Autodesk Inventor part; units mm, degrees
ref_plane "YZ Plane" through (0, 0, 0) normal (1, 0, 0) x (0, 1, 0)
ref_plane "XZ Plane" through (0, 0, 0) normal (0, 1, 0) x (-1, 0, 0)
ref_plane "XY Plane" through (0, 0, 0) normal (0, 0, 1) x (1, 0, 0)
sketch "Sketch1" plane through (0, 0, 0) normal (0, 1, 0) x (-1, 0, 0)
  line L0 (0, 0) -> (145, 0)
  line L1 (145, 0) -> (145, -145)
  line L2 (145, -145) -> (0, -145)
  line L3 (0, -145) -> (0, 0)
  dimension "d0" = 145
  dimension "d1" = 145
extrude "Extrusion1" add sketch "Sketch1" along normal blind 5
sketch "Sketch2" plane through (0, 5, 0) normal (0, 1, 0) x (1, 0, 0)
  line L0 (-145, 145) -> (-145, 0)
  line L1 (0, 145) -> (-145, 145)
  point P0 (0, 0)
  point P1 (-140, 72.5)
  dimension "d4" = 5
  dimension "d5" = 72.5
hole "Hole1" at (-140, 5, -72.5) direction (0, -1, 0) diameter 4 end through all
sketch "Sketch3" plane through (0, 5, 0) normal (0, 1, 0) x (1, 0, 0)
  line L0 (0, 0) -> (0, 145)
  line L1 (0, 145) -> (-145, 145)
  point P0 (-5, 72.5)
  dimension "d13" = 5
  dimension "d14" = 72.5
hole "Hole2" at (-5, 5, -72.5) direction (0, -1, 0) diameter 4 end through all
properties part number "pot_mover"
Build history of the part. All positions in model axes, mm. Round coordinates to 2 decimals unless told otherwise and drop trailing zeros. Loops run counter-clockwise (first coordinate to the right, second up) from the corner with the lowest first, then second, coordinate; pieces in that order, holes last.
Item 1: Saw through at B-B (z = -72.5). List the corners of the cut face in (x, y), then the cut area to 3 significant figures.
Item 2: Saw through at A-A (x = -5). List the corners of the cut face in (y, z), then the cut area to 3 significant figures.
Item 3: Drill centre lines: line 1 along X through (y, z) = (2.65, -72.5); line 2 along Z through (x, y) = (-140, 1.25). Where is each one in solid material? Low to high.
Item 4: Two-plate mould, pull along X, no slides. Class faces 1 (the face through (-145, 2, -71)), 2 (the face through (-71, 0, -71)), 3 (the face through (-138.226, 2.465, -71.577)): released by +X, released by -X, zero draft, split by the parting line, or undercut.
Item 5: Pin check, flat tip, straight feed: P1, Ø3, axis at x = -129.5, y = 3, coming from the +Z side. Stop position of the tip, or through.
Worked answers:
1. outline: (-145, 0) - (-142, 0) - (-142, 5) - (-145, 5) - close; (-138, 0) - (-7, 0) - (-7, 5) - (-138, 5) - close; (-3, 0) - (0, 0) - (0, 5) - (-3, 5) - close
1. area: 685 mm2
2. outline: (0, -145) - (5, -145) - (5, -74.5) - (0, -74.5) - close; (0, -70.5) - (5, -70.5) - (5, 0) - (0, 0) - close
2. area: 705 mm2
3. line 1: x = -145 to -142, -138 to -7, -3 to 0
3. line 2: z = -145 to -74.5, -70.5 to 0
4. face 1: released by -X
4. face 2: zero draft
4. face 3: undercut
5. P1: stops at z = 0
